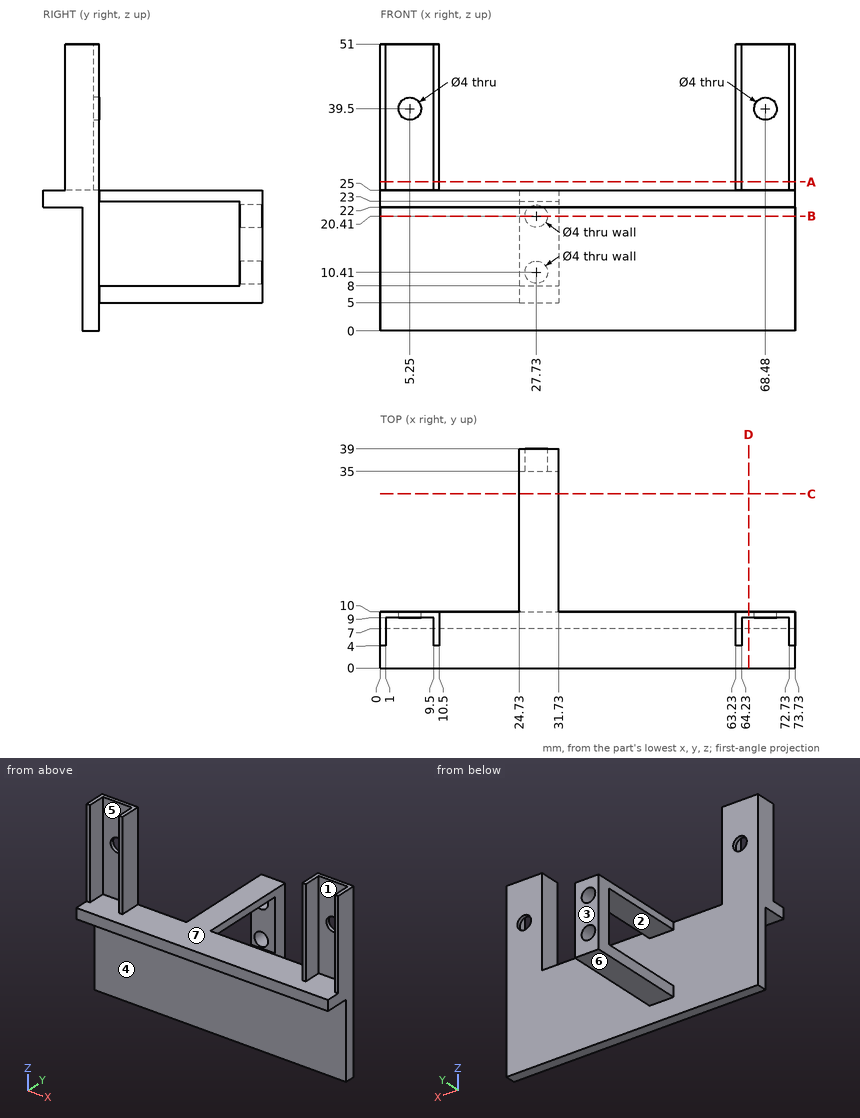
Design review of the part shown in the three views and the two pictorial views. Dimensions are in mm from the part's minimum x, y and z. A direction names the side the tool comes from. Coordinates: 2 decimals unless noted, no trailing zeros. Write each loop counter-clockwise with the first axis right and the second up, starting at its lowest first coordinate (ties: lowest second). Pieces come first, ordered by that corner, then holes.
(1) The part is to be moulded in two halves that separate along X. For the marked faces 5, 6 and 7, say which applies: +X half, -X half, draft (parallel to the pull), parting line (faces both ways), or undercut.
(2) Add section A-A on z = 26.5. Give the boundary of the cut face in (x, y), then the cut area to 3 significant figures.
(3) Add section D-D on x = 65.5. Give the boundary of the cut face in (y, z), then the cut area to 3 significant figures.
(4) Add section C-C on y = 31. Give the boundary of the cut face in (x, z), then the cut area to 3 significant figures.
(5) For pin 1 Ø3.5 at (x, z) = (28.5, 12) entering from -Y; pin 2 Ø7 at (x, z) = (4, 35) entering from -Y; pin 3 Ø12 at (y, z) = (33.5, 16) entering from -X, all flat-tipped, find the tip position at first contact; note any pin that passes through.
(6) Add section B-B on z = 20.41. Give the boundary of the cut face in (x, y).
(7) Wall thickness on probe 1 along X at (y, z) = (9.2, 39.5); probe 2 along X at (y, z) = (5.5, 30.5); probe 3 along X at (y, z) = (36.7, 20.41): over which ranges is each line inside the solid? List them lowest first.
(8) Tool access review of the marked faces 1, 2, 3 and 4: name each direction out of +Z, -Z, +X, -X, +Y, -Y from which nothing blocks a thin tool from reaching the whole face with its end or side.
Answer sheet:
1. face 5: undercut
1. face 6: draft
1. face 7: undercut
2. outline: (0, 4) - (1, 4) - (1, 9) - (9.5, 9) - (9.5, 4) - (10.5, 4) - (10.5, 10) - (0, 10) - close; (63.23, 4) - (64.23, 4) - (64.23, 9) - (72.73, 9) - (72.73, 4) - (73.73, 4) - (73.73, 10) - (63.23, 10) - close
2. area: 41.0 mm2
3. outline: (0, 22) - (7, 22) - (7, 0) - (10, 0) - (10, 51) - (9, 51) - (9, 25) - (0, 25) - close
3. area: 122 mm2
4. outline: (24.73, 5) - (31.73, 5) - (31.73, 8) - (24.73, 8) - close; (24.73, 23) - (31.73, 23) - (31.73, 25) - (24.73, 25) - close
4. area: 35.0 mm2
5. pin 1: stops at y = 7
5. pin 2: stops at y = 4
5. pin 3: stops at x = 24.73
6. outline: (0, 7) - (73.73, 7) - (73.73, 10) - (0, 10) - close; (24.73, 35) - (25.73, 35) - (25.73, 39) - (24.73, 39) - close; (29.73, 35) - (31.73, 35) - (31.73, 39) - (29.73, 39) - close
7. probe 1: x = 0 to 3.25, 7.25 to 10.5, 63.23 to 66.48, 70.48 to 73.73
7. probe 2: x = 0 to 1, 9.5 to 10.5, 63.23 to 64.23, 72.73 to 73.73
7. probe 3: x = 24.73 to 25.73, 29.73 to 31.73
8. face 1: +Z, -Y
8. face 2: +X, -X
8. face 3: +Z, -Z, +X, -X, +Y
8. face 4: -Z, +X, -X, -Y
